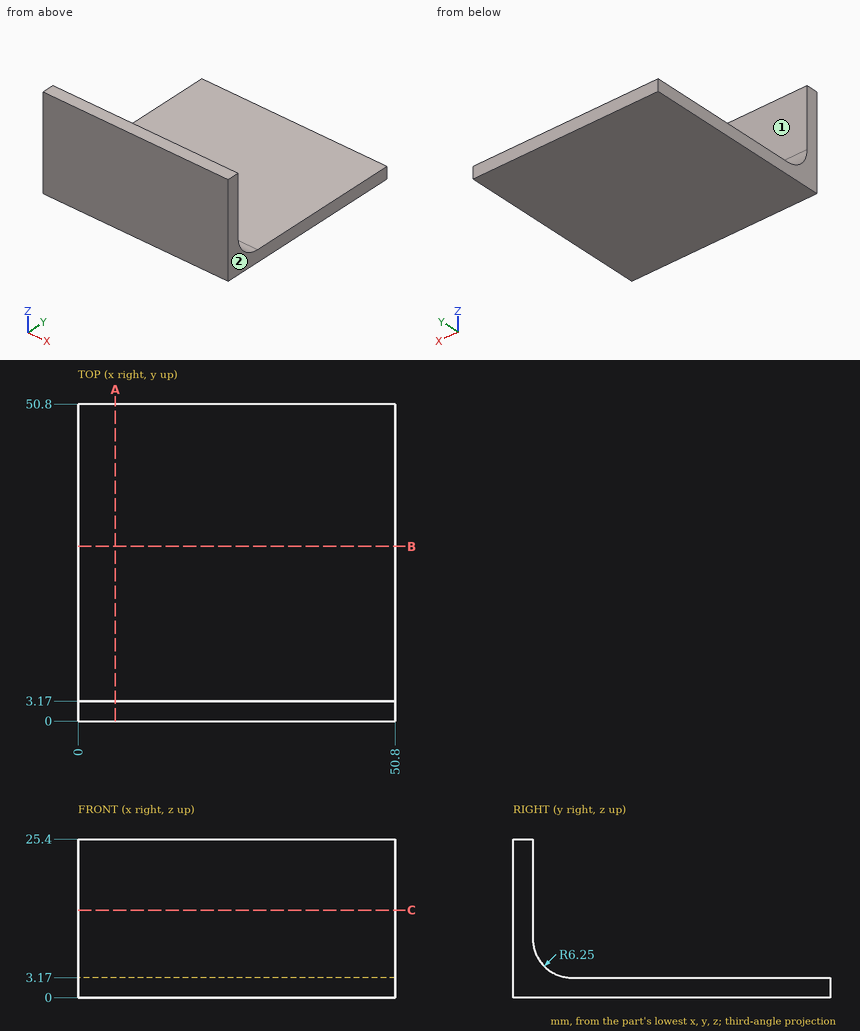
Source: three-view drawing plus pictorial views. Frame: mm from the lowest corner of the part. A direction names the side the tool comes from. Round coordinates to 2 decimals unless told otherwise and drop trailing zeros. Loops run counter-clockwise (first coordinate to the right, second up) from the corner with the lowest first, then second, coordinate; pieces in that order, holes last. Notation, with made-up numbers: (-32.5, 75) - (-10.5, 75) arc R16 ccw to (-10.5, 106) - close; hole circle Ø9 at (-23, 77). An arc over 180 degrees is marked (long way). Write each question's results on one line, items separated by ' | '. Start each with the question number.
1) Cut plane A-A on x = 6. Return loops of the section in (y, z).
2) Line query: probe 1 along Z at (x, y) = (12.5, 47.5); probe 2 along Y at (x, z) = (14, 9); probe 3 along Y at (x, z) = (40.5, 7.5). Output: solid intervals per line, ascending. Write a range as [from, to].
3) First-contact query: P1, Ø1, axis at x = 7, y = 12.5, coming from the +Z side; P2, Ø13, axis at x = 21, z = 18.5, coming from the +Y side; P3, Ø1.5, axis at x = 6, y = 7, coming from the +Z side; P4, Ø8, axis at x = 20, z = 3.5, coming from the +Y side. Flat tips, straight axial feed; report the tip coordinate or a pass-through.
4) Access query for the marked faces 1 and 2. Directions: +Z, -Z, +X, -X, +Y, -Y. A direction counts if a zero-diameter tool reaches every point of the face in a straight line with its end or side. Return the directions, or none.
5) Cut plane B-B on y = 28. Return loops of the section in (x, z).
Verdict:
1) outline: (0, 0) - (50.8, 0) - (50.8, 3.17) - (9.42, 3.17) arc R6.25 cw to (3.17, 9.42) - (3.17, 25.4) - (0, 25.4) - close
2) probe 1: z = [0, 3.17] | probe 2: y = [0, 3.18] | probe 3: y = [0, 3.47]
3) P1: stops at z = 3.17 | P2: stops at y = 3.17 | P3: stops at z = 4.03 | P4: stops at y = 50.8
4) face 1: +Z, +X, -X, +Y | face 2: +Z, -Z, +X, +Y, -Y
5) outline: (0, 0) - (50.8, 0) - (50.8, 3.17) - (0, 3.17) - close
